The listing builds one solid part. Answer for the finished solid, in the listing's coordinates (mm). A direction names the side the tool comes from. Round coordinates to 2 decimals unless told otherwise and drop trailing zeros. Order: outer loops, then holes, each group sorted by start corner. A loop starts at its lowest first (then second) coordinate and runs counter-clockwise, first axis right, second up. Notation, with made-up numbers: (37.25, 73) - (82.25, 73) arc R24 ccw to (82.25, 106) - close; hole circle Ø7 at (17.25, 4). An arc over 180 degrees is marked (long way). Use CSV: the item, a comma, the result in double quotes. Start each with the question number.
Item 1: Flat-ended cylindrical pins translate along their axes: P1, Ø8, axis at y = 1, z = 6.5, coming from the -X side; P2, Ø8, axis at x = 4.5, z = 17, coming from the +Y side; P3, Ø5, axis at x = -14, y = 9, coming from the -Z side; P4, Ø5, axis at x = 18.5, y = 4, coming from the +Z side. Find the tip coordinate at first contact, or state that the pin passes through.
Item 2: Find section B-B, the plane y = 0. Count the separate pieces of the cut face and the enclosed holes in it, plus the area to 3 significant figures.
Item 3: For faces 1 (the flat face through (0, 0, 0)), 2 (the flat face through (-14.5, 4.8, 1.3)), determine the directions among +Z, -Z, +X, -X, +Y, -Y from which every point of the face is accessible in a straight line to the end or side of a thin tool.
Item 4: Straight lines are drawn through the part: line 1 along Z through (x, y) = (-15, 2.5); line 2 along Z through (x, y) = (6.5, 5.5); line 3 along Y through (x, z) = (-19.35, 1). For each, find the intervals that lie inside material, in ascending order. Write a range as [from, to].
Item 5: Find section A-A, the plane x = 19.35. Give the vertices of the cut face in (y, z).
Item 6: Find section D-D, the plane z = 16.5. Give the vertices of the cut face in (x, y).
Item 7: Find section C-C, the plane z = 4.25. Give the vertices of the cut face in (x, y), plus the area to 3 significant figures.
```python
from build123d import *

# Parameters (mm, degrees)
F0_R     = 2.1
F0_R_2   = 14.15
F0_R_3   = 10.3
F0_R_4   = 7.1
F1_DEPTH = 1.3
F2_DEPTH = 14.05
F3_DEPTH = 15.95
F4_R     = 0.9
F6_R     = 0.4
F7_R     = 1


# Not quite as in the source:
# - a fillet or chamfer that OpenCascade refuses, or shapes differently, is made with other operations: its cross-section is extruded or revolved along the edge and cut away or added


with BuildPart() as f1:
    # F0 (on Top) → F1 (new body)
    with BuildSketch(Plane.XY):
        with BuildLine():
            Line((9.1782945736, -13.1056823065), (22.1608527132, -4.0136152064))
            ThreePointArc((22.1608527132, -4.0136152064), (24.25, 0), (22.1608527132, 4.0136152064))
            Line((22.1608527132, 4.0136152064), (9.1782945736, 13.1056823065))
            ThreePointArc((9.1782945736, 13.1056823065), (0, 16), (-9.1782945736, 13.1056823065))
            Line((-9.1782945736, 13.1056823065), (-22.1608527132, 4.0136152064))
            ThreePointArc((-22.1608527132, 4.0136152064), (-24.25, 0), (-22.1608527132, -4.0136152064))
            Line((-22.1608527132, -4.0136152064), (-9.1782945736, -13.1056823065))
            ThreePointArc((-9.1782945736, -13.1056823065), (0, -16), (9.1782945736, -13.1056823065))
        make_face()
        with Locations((-19.35, 0)):
            Circle(F0_R, mode=Mode.SUBTRACT)
        Circle(F0_R_2, mode=Mode.SUBTRACT)
        with Locations((19.35, 0)):
            Circle(F0_R, mode=Mode.SUBTRACT)
        Circle(F0_R_2)
        Circle(F0_R_3, mode=Mode.SUBTRACT)
        Circle(F0_R_3)
        Circle(F0_R_4, mode=Mode.SUBTRACT)
        Circle(F0_R_4)
    extrude(amount=F1_DEPTH)

    # F0 (on Top) → F2 (join)
    with BuildSketch(Plane.XY):
        Circle(F0_R_2)
        Circle(F0_R_3, mode=Mode.SUBTRACT)
        Circle(F0_R_3)
        Circle(F0_R_4, mode=Mode.SUBTRACT)
        Circle(F0_R_4)
    extrude(amount=F2_DEPTH)

    # F0 (on Top) → F3 (join)
    with BuildSketch(Plane.XY):
        Circle(F0_R_3)
        Circle(F0_R_4, mode=Mode.SUBTRACT)
    extrude(amount=F3_DEPTH)

    # F4
    f4_edges = [f1.edges().sort_by_distance(p)[0] for p in [
        (-14.15, 0, 1.3),
    ]]
    fillet(f4_edges, radius=F4_R)

    # F5: fillet of radius 9 on 1 edges, made by hand

    # F5_s1 → F5_t2 (revolve, cut)
    with BuildSketch(Plane.XZ):
        with BuildLine():
            ThreePointArc((14.15, 6.6691125195), (13.129661647, 10.8314435971), (10.3, 14.05))
            Line((10.3, 14.05), (14.15, 14.05))
            Line((14.15, 14.05), (14.15, 6.6691125195))
        make_face()
    revolve(axis=Axis((0, 0, 14.05), (0, 0, 1)), mode=Mode.SUBTRACT)

    # F6
    f6_edges = [f1.edges().sort_by_distance(p)[0] for p in [
        (-10.3, 0, 14.05),
    ]]
    fillet(f6_edges, radius=F6_R)

    # F7
    f7_edges = [f1.edges().sort_by_distance(p)[0] for p in [
        (-10.3, 0, 15.95),
        (-7.1, 0, 15.95),
    ]]
    fillet(f7_edges, radius=F7_R)

    # F9 (on offset) → F10 (revolve)
    with BuildSketch(Plane.XY.offset(11.35)):
        with BuildLine():
            Line((0, -8), (0, 8))
            ThreePointArc((0, 8), (-8, 0), (0, -8))
        make_face()
    revolve(axis=Axis((0, -0.0622457136, 11.35), (0, 1, 0)))


solid = f1.part
```
Worked out:
1,P1,"stops at x = -14.15"
1,P2,"stops at y = 10.87"
1,P3,"stops at z = 0"
1,P4,"stops at z = 1.3"
2,separate pieces,"3"
2,enclosed holes,"0"
2,area,"465 mm²"
3,face 1,"-Z, +X, -X, +Y, -Y"
3,face 2,"+Z"
4,line 1,"z = [0, 1.3]"
4,line 2,"z = [0, 15.95]"
4,line 3,"y = [-5.98, -2.1], [2.1, 5.98]"
5,outline,"(-5.98, 0) - (-2.1, 0) - (-2.1, 1.3) - (-5.98, 1.3) - close; (2.1, 0) - (5.98, 0) - (5.98, 1.3) - (2.1, 1.3) - close"
6,outline,"circle Ø12.24 at (0, 0)"
7,outline,"circle Ø28.3 at (0, 0)"
7,area,"629 mm²"
